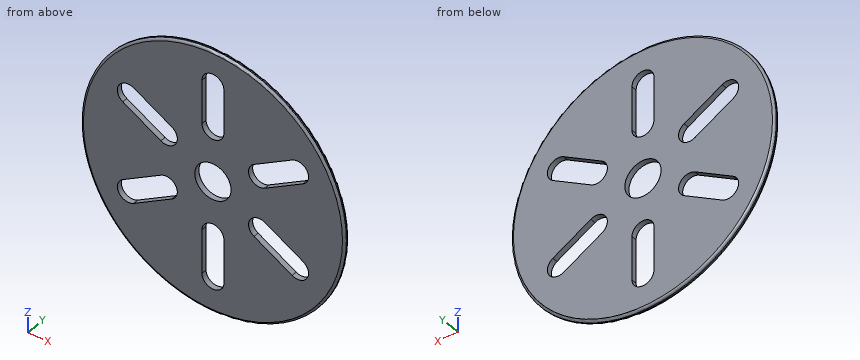
```python
from build123d import *

# Parameters (mm, degrees)
F0_R     = 304.8
F0_R_2   = 41.91
F1_DEPTH = 12.7
F3_DEPTH = 12.701
F4_R     = 5.08


# Not quite as in the source:
# - a feature names something its author has since deleted; it is built from what else it names


with BuildPart() as f1:
    # F0 (on Front) → F1 (new body)
    with BuildSketch(Plane.XZ):
        Circle(F0_R)
        Circle(F0_R_2, mode=Mode.SUBTRACT)
    extrude(amount=F1_DEPTH)

    # F2 (on face) → F3 (cut, through all)
    with BuildSketch(Plane.XZ.offset(12.7)):
        with BuildLine():
            Line((-25.4, 226.06), (-25.4, 124.46))
            ThreePointArc((-25.4, 124.46), (0, 99.06), (25.4, 124.46))
            Line((25.4, 124.46), (25.4, 226.06))
            ThreePointArc((25.4, 226.06), (0, 251.46), (-25.4, 226.06))
        make_face()
        with BuildLine():
            Line((-183.0737027795, -135.0270452561), (-95.085521755, -84.2270452561))
            ThreePointArc((-95.085521755, -84.2270452561), (-85.7884764989, -49.53), (-120.485521755, -40.2329547439))
            Line((-120.485521755, -40.2329547439), (-208.4737027795, -91.0329547439))
            ThreePointArc((-208.4737027795, -91.0329547439), (-217.7707480356, -125.73), (-183.0737027795, -135.0270452561))
        make_face()
        with BuildLine():
            Line((-208.4737027795, 91.0329547439), (-120.485521755, 40.2329547439))
            ThreePointArc((-120.485521755, 40.2329547439), (-85.7884764989, 49.53), (-95.085521755, 84.2270452561))
            Line((-95.085521755, 84.2270452561), (-183.0737027795, 135.0270452561))
            ThreePointArc((-183.0737027795, 135.0270452561), (-217.7707480356, 125.73), (-208.4737027795, 91.0329547439))
        make_face()
        with BuildLine():
            Line((183.0737027795, 135.0270452561), (95.085521755, 84.2270452561))
            ThreePointArc((95.085521755, 84.2270452561), (85.7884764989, 49.53), (120.485521755, 40.2329547439))
            Line((120.485521755, 40.2329547439), (208.4737027795, 91.0329547439))
            ThreePointArc((208.4737027795, 91.0329547439), (217.7707480356, 125.73), (183.0737027795, 135.0270452561))
        make_face()
        with BuildLine():
            Line((208.4737027795, -91.0329547439), (120.485521755, -40.2329547439))
            ThreePointArc((120.485521755, -40.2329547439), (85.7884764989, -49.53), (95.085521755, -84.2270452561))
            Line((95.085521755, -84.2270452561), (183.0737027795, -135.0270452561))
            ThreePointArc((183.0737027795, -135.0270452561), (217.7707480356, -125.73), (208.4737027795, -91.0329547439))
        make_face()
        with BuildLine():
            Line((25.4, -226.06), (25.4, -124.46))
            ThreePointArc((25.4, -124.46), (0, -99.06), (-25.4, -124.46))
            Line((-25.4, -124.46), (-25.4, -226.06))
            ThreePointArc((-25.4, -226.06), (0, -251.46), (25.4, -226.06))
        make_face()
    extrude(amount=-F3_DEPTH, mode=Mode.SUBTRACT)

    # F4
    f4_edges = [f1.edges().sort_by_distance(p)[0] for p in [
        (-304.8, 0, 0),
        (-304.8, -12.7, 0),
    ]]
    fillet(f4_edges, radius=F4_R)


solid = f1.part
```
CAD build for the part. Positions are in the model's coordinates, mm. Round coordinates to 2 decimals unless told otherwise and drop trailing zeros. Order: outer loops, then holes, each group sorted by start corner. A loop starts at its lowest first (then second) coordinate and runs counter-clockwise, first axis right, second up.
Q1. Slice it at B-B (z = 0). Write the cut outline in (x, y), and give its area (3 significant figures).
Q2. Slice it at A-A (x = 0). Write the cut outline in (y, z).
Q3. Wall check: L1, parallel to Z at x = 0, y = -8.5; L2, parallel to Z at x = 0, y = -4.75; L3, parallel to Z at x = -192, y = -5.75. Give the ranges that are in metal, low to high.
Q4. Drop flat-ended pins along their axis: pin 1 (3 mm diameter, centred on x = 87.5, y = -4.5, fed in from +Z); pin 2 (5 mm diameter, centred on x = -222.5, y = -8.5, fed in from +Z); pin 3 (1 mm diameter, centred on y = -2.5, z = 29, fed in from -X); pin 4 (2 mm diameter, centred on x = 38, z = -201.5, fed in from +Y). Give the stop position or say it passes through.
Q5. Slice it at C-C (z = -113.03). State how many separate pieces and enclosed holes the cut face has, and give its area (3 significant figures).
Results below:
1. outline: (-304.8, -7.62) arc R5.08 ccw to (-299.72, -12.7) - (-41.91, -12.7) - (-41.91, 0) - (-299.72, 0) arc R5.08 ccw to (-304.8, -5.08) - close; (41.91, -12.7) - (299.72, -12.7) arc R5.08 ccw to (304.8, -7.62) - (304.8, -5.08) arc R5.08 ccw to (299.72, 0) - (41.91, 0) - close
1. area: 6,660 mm2
2. outline: (-12.7, -299.72) arc R5.08 ccw to (-7.62, -304.8) - (-5.08, -304.8) arc R5.08 ccw to (0, -299.72) - (0, -251.46) - (-12.7, -251.46) - close; (-12.7, -99.06) - (0, -99.06) - (0, -41.91) - (-12.7, -41.91) - close; (-12.7, 41.91) - (0, 41.91) - (0, 99.06) - (-12.7, 99.06) - close; (-12.7, 251.46) - (0, 251.46) - (0, 299.72) arc R5.08 ccw to (-5.08, 304.8) - (-7.62, 304.8) arc R5.08 ccw to (-12.7, 299.72) - close
3. L1: z = -304.72 to -251.46, -99.06 to -41.91, 41.91 to 99.06, 251.46 to 304.72
3. L2: z = -304.79 to -251.46, -99.06 to -41.91, 41.91 to 99.06, 251.46 to 304.79
3. L3: z = -236.73 to -138.15, -81.52 to 81.52, 138.15 to 236.73
4. pin 1: stops at z = 292.4
4. pin 2: stops at z = 210.89
4. pin 3: stops at x = -302.97
4. pin 4: stops at y = 0
5. separate pieces: 4
5. enclosed holes: 0
5. area: 4,650 mm2
